Verification items for the finished model (mm, model axes). A direction names the side the tool comes from. Give positions to 0.01 mm unless a question says otherwise; leave off trailing zeros. Write each loop counter-clockwise with the first axis right and the second up, starting at its lowest first coordinate (ties: lowest second). Pieces come first, ordered by that corner, then holes. Notation, with made-up numbers: (35.5, -36) - (43.5, -36) arc R12 ccw to (43.5, -14) - close; hole circle Ø7 at (25.5, 56). An arc over 180 degrees is marked (long way). Answer as a JSON object with one key per item and string values. Group by question number.
Item 1: Sectioned sample at B-B, the plane x = 10. Record the boundary of the cut face in (y, z), and give its area (3 significant figures).
Item 2: Sectioned sample at A-A, the plane y = 14.5. Record the boundary of the cut face in (x, z), and give its area (3 significant figures).
Item 3: Tool access check on faces 1 (the face through (48.26, 23, 3)), 2 (the face through (30, 35, 0)), 3 (the face through (67, 40.894, 18)), 4 (the face through (62, 6.35, 8)). Record the directions out of +Z, -Z, +X, -X, +Y, -Y that give a thin tool (end or side, any length) a straight path to the whole face; none if there is none.
Item 4: Draft check along X on faces 5 (the face through (24, 40.894, 3)), 6 (the face through (2.6, 17.71, 2.58)), 7 (the face through (60.743, 23.645, 8.938)). Enter one of: +X half, -X half, draft (parallel to the pull), parting line (faces both ways), or undercut.
Item 5: Scan lines: line 1 along Y through (x, z) = (68.05, 22.86); line 2 along X through (y, z) = (31, 2); line 3 along X through (y, z) = (6, 5.75). Record each from-to range of solid material in increasing order. Write a range as [from, to].
Item 6: Sectioned sample at D-D, the plane y = 38. Record the boundary of the cut face in (x, z).
Item 7: Sectioned sample at C-C, the plane z = 2.5. Record the boundary of the cut face in (x, y) (3 decimals).
Item 8: Go/stop test with flat-tipped pins: pin 1 (1.5 mm diameter, centred on y = 34.417, z = 22.86, fed in from -X); pin 2 (5 mm diameter, centred on x = 18, z = 6.5, fed in from -Y); pin 3 (4 mm diameter, centred on x = 16.5, z = 5, fed in from +Y). Record where each tip stops, or that it passes through.
```python
from build123d import *

# Parameters (mm, degrees)
SKETCH1_W            = 54.61
SKETCH1_H            = 47.244
SKETCH1_W_2          = 41.91
SKETCH1_H_2          = 21.844
BOSS_EXTRUDE1_DEPTH  = 5.08
SKETCH2_R            = 0.93599
CUT_EXTRUDE1_DEPTH   = 73.388217522
SKETCH10_W           = 14.41958
SKETCH10_H           = 19.49958
SKETCH10_R           = 0.635
BOSS_EXTRUDE4_DEPTH  = 5.08
SKETCH11_R           = 0.635
SKETCH11_W           = 3.302
SKETCH11_H           = 76.2
BOSS_EXTRUDE5_DEPTH  = 5.08
SKETCH12_W           = 60.452
SKETCH12_H           = 6.35
SKETCH12_W_2         = 59.182
CUT_EXTRUDE2_DEPTH   = 95.448366629
SKETCH13_W           = 7.0195552
SKETCH13_H           = 78.993394517
BOSS_EXTRUDE6_DEPTH  = 4.826
FILLET1_R            = 2.54
CUT_EXTRUDE3_DEPTH   = 95.448366629
SKETCH15_W           = 9.078627065
SKETCH15_H           = 34.544
BOSS_EXTRUDE7_DEPTH  = 5.08
SKETCH19_W           = 25.4
SKETCH19_H           = 34.544
BOSS_EXTRUDE9_DEPTH  = 4.7625
SKETCH20_W           = 9.525
SKETCH20_H           = 9.525
BOSS_EXTRUDE10_DEPTH = 9.525
SKETCH21_R           = 0.635
CUT_EXTRUDE4_DEPTH   = 98.23065776
SKETCH22_R           = 0.635
CUT_EXTRUDE5_DEPTH   = 98.23065776
RIB1_REACH           = 80.493
SKETCH24_WALL_W      = 169.76250031
SKETCH24_WALL_H      = 2.54
FILLET2_R            = 1.27


with BuildPart() as part:
    # Sketch1 → Boss-Extrude1 (new body)
    with BuildSketch(Plane.XY):
        with Locations((27.305, 23.622)):
            Rectangle(SKETCH1_W, SKETCH1_H)
        with Locations((27.305, 23.622)):
            Rectangle(SKETCH1_W_2, SKETCH1_H_2, mode=Mode.SUBTRACT)
    extrude(amount=BOSS_EXTRUDE1_DEPTH)

    # Sketch2 → Cut-Extrude1 (cut, through all)
    with BuildSketch(Plane.XY.offset(5.08)):
        with Locations((2.80543, 28.62199)):
            Circle(SKETCH2_R)
        with Locations((2.80543, 18.62201)):
            Circle(SKETCH2_R)
        with Locations((51.80457, 28.62199)):
            Circle(SKETCH2_R)
        with Locations((51.80457, 18.62201)):
            Circle(SKETCH2_R)
    extrude(amount=-CUT_EXTRUDE1_DEPTH, mode=Mode.SUBTRACT)

    # Sketch10 → Boss-Extrude4 (add)
    with BuildSketch(Plane.XY.offset(5.08)):
        with Locations((61.81979, 23.622)):
            Rectangle(SKETCH10_W, SKETCH10_H)
        with Locations((64.35979, 21.49221)):
            Circle(SKETCH10_R, mode=Mode.SUBTRACT)
        with Locations((64.35979, 25.75179)):
            Circle(SKETCH10_R, mode=Mode.SUBTRACT)
    extrude(amount=-BOSS_EXTRUDE4_DEPTH)

    # Sketch11 → Boss-Extrude5 (add)
    with BuildSketch(Plane.XY.offset(5.08)):
        Polygon((0, 47.244), (-5.842, 47.244), (-5.842, 64.262), (-15.748, 64.262), (-15.748, -17.018), (-4.572, -17.018), (-4.572, 0), (0, 0), align=None)
        with Locations(Location((-4.572, 21.49221, 0), (0, 0, 180))):
            Circle(SKETCH11_R, mode=Mode.SUBTRACT)
        with Locations(Location((-4.572, 25.75179, 0), (0, 0, 180))):
            Circle(SKETCH11_R, mode=Mode.SUBTRACT)
        with Locations((-10.795, 23.622)):
            Rectangle(SKETCH11_W, SKETCH11_H, mode=Mode.SUBTRACT)
    extrude(amount=-BOSS_EXTRUDE5_DEPTH)

    # Sketch12 → Cut-Extrude2 (cut, through all)
    with BuildSketch(Plane.XY.offset(5.08)):
        with Locations((24.384, 44.069)):
            Rectangle(SKETCH12_W, SKETCH12_H)
        with Locations((25.019, 3.175)):
            Rectangle(SKETCH12_W_2, SKETCH12_H)
    extrude(amount=-CUT_EXTRUDE2_DEPTH, mode=Mode.SUBTRACT)

    # Sketch13 → Boss-Extrude6 (add)
    with BuildSketch(Plane(origin=(0, 0, 0), x_dir=(-1, 0, 0), z_dir=(0, 0, -1))):
        with Locations((10.665198327, 23.388014827)):
            Rectangle(SKETCH13_W, SKETCH13_H)
    extrude(amount=-BOSS_EXTRUDE6_DEPTH)

    # Fillet1
    fillet1_edges = [part.edges().sort_by_distance(p)[0] for p in [
        (69.02958, 13.87221, 2.54),
        (54.61, 13.87221, 2.54),
        (54.61, 6.35, 2.54),
        (-4.572, 6.35, 2.54),
        (-4.572, -17.018, 2.54),
        (-15.748, -17.018, 2.54),
        (-15.748, 64.262, 2.54),
        (-5.842, 64.262, 2.54),
        (-5.842, 40.894, 2.54),
        (54.61, 40.894, 2.54),
        (54.61, 33.37179, 2.54),
        (69.02958, 33.37179, 2.54),
    ]]
    fillet(fillet1_edges, radius=FILLET1_R)

    # Sketch14 → Cut-Extrude3 (cut, through all)
    with BuildSketch(Plane.XY.offset(5.08)):
        Polygon((2.80543, 40.894), (-0.815942935, 40.894), (-0.815942935, 6.35), (2.80543, 6.35), (2.80543, -19.941776761), (-23.515321153, -19.941776761), (-23.515321153, 65.826532556), (2.80543, 65.826532556), align=None)
        Polygon((51.80457, 40.896870143), (51.80457, 65.826532556), (74.486186006, 65.826532556), (74.486186006, -19.941776761), (51.80457, -19.941776761), (52.07, 6.35), (54.61, 8.89), (54.61, 38.354), align=None)
    extrude(amount=-CUT_EXTRUDE3_DEPTH, mode=Mode.SUBTRACT)

    # Sketch15 → Boss-Extrude7 (add)
    with BuildSketch(Plane.XY.offset(5.08)):
        with Locations((-5.355256468, 23.622)):
            Rectangle(SKETCH15_W, SKETCH15_H)
        Polygon((51.807736495, 40.894), (54.61, 38.354), (54.61, 8.89), (52.07, 6.35), (64.50457, 6.35), (64.50457, 40.894), align=None)
    extrude(amount=-BOSS_EXTRUDE7_DEPTH)

    # Sketch19 → Boss-Extrude9 (add)
    with BuildSketch(Plane(origin=(64.50457, 0, 0), x_dir=(0, 0, -1), z_dir=(1, 0, 0))):
        with Locations((-12.7, 23.622)):
            Rectangle(SKETCH19_W, SKETCH19_H)
    extrude(amount=BOSS_EXTRUDE9_DEPTH)

    # Sketch20 → Boss-Extrude10 (add)
    with BuildSketch(Plane(origin=(69.26707, 0, 0), x_dir=(0, 0, -1), z_dir=(1, 0, 0))):
        with Locations((-4.7625, 45.6565)):
            Rectangle(SKETCH20_W, SKETCH20_H)
        with Locations((-4.7625, 1.5875)):
            Rectangle(SKETCH20_W, SKETCH20_H)
    extrude(amount=-BOSS_EXTRUDE10_DEPTH)

    # Sketch21 → Cut-Extrude4 (cut, through all)
    with BuildSketch(Plane(origin=(69.26707, 0, 0), x_dir=(0, 0, -1), z_dir=(1, 0, 0))):
        with Locations((-4.7625, 45.6565)):
            Circle(SKETCH21_R)
        with Locations((-4.7625, 1.5875)):
            Circle(SKETCH21_R)
    extrude(amount=-CUT_EXTRUDE4_DEPTH, mode=Mode.SUBTRACT)

    # Sketch22 → Cut-Extrude5 (cut, through all)
    with BuildSketch(Plane(origin=(69.26707, 0, 0), x_dir=(0, 0, -1), z_dir=(1, 0, 0))):
        with Locations((-22.86, 34.417)):
            Circle(SKETCH22_R)
        with Locations((-22.86, 12.827)):
            Circle(SKETCH22_R)
        with Locations((-16.51, 34.417)):
            Circle(SKETCH22_R)
        with Locations((-10.16, 34.417)):
            Circle(SKETCH22_R)
        with Locations((-10.16, 12.827)):
            Circle(SKETCH22_R)
        with Locations((-16.51, 12.827)):
            Circle(SKETCH22_R)
    extrude(amount=-CUT_EXTRUDE5_DEPTH, mode=Mode.SUBTRACT)

    # Sketch24 wall → Rib1 (add, up to next)
    with BuildSketch(Plane(origin=(60.69457, 23.622, 8.89), x_dir=(-0.707106781187, 0, -0.707106781187), z_dir=(0.707106781187, 0, -0.707106781187)), mode=Mode.PRIVATE) as rib1_sk1:
        Rectangle(SKETCH24_WALL_W, SKETCH24_WALL_H)
    rib1_tool1 = extrude(rib1_sk1.sketch, amount=RIB1_REACH, mode=Mode.PRIVATE) - part.part
    add(rib1_tool1.solids().sort_by_distance((60.69457, 23.622, 8.89))[0])

    # Fillet2
    fillet2_edges = [part.edges().sort_by_distance(p)[0] for p in [
        (62.12332, 6.35, 5.08),
        (64.50457, 14.351, 5.08),
        (66.88582, 40.894, 25.4),
        (66.88582, 6.35, 25.4),
        (62.12332, 40.894, 5.08),
        (66.88582, 40.894, 9.525),
        (66.88582, 6.35, 9.525),
        (64.50457, 32.893, 5.08),
        (64.50457, 23.622, 12.7),
        (56.88457, 23.622, 5.08),
        (60.69457, 22.352, 5.08),
        (60.69457, 24.892, 5.08),
    ]]
    fillet(fillet2_edges, radius=FILLET2_R)


solid = part.part
```
Geometry check:
{
 "1": {"outline": "(6.35, 0) - (12.7, 0) - (12.7, 5.08) - (6.35, 5.08) - close; (34.54, 0) - (40.89, 0) - (40.89, 5.08) - (34.54, 5.08) - close", "area": "64.5 mm^2"},
 "2": {"outline": "(-9.89, 0) - (6.35, 0) - (6.35, 5.08) - (-9.89, 5.08) - close; (48.26, 0) - (69.27, 0) - (69.27, 25.4) - (64.5, 25.4) - (64.5, 6.35) arc R1.27 cw to (63.23, 5.08) - (48.26, 5.08) - close", "area": "286 mm^2"},
 "3": {"face 1": "+Z, -Z", "face 2": "-Z, +X, -X, +Y, -Y", "face 3": "+Z, +X, -X, +Y", "face 4": "+Z, -X"},
 "4": {"face 5": "draft", "face 6": "undercut", "face 7": "-X half"},
 "5": {"line 1": "[6.35, 12.19], [13.46, 33.78], [35.05, 40.89]", "line 2": "[-9.89, 6.35], [48.26, 69.27]", "line 3": "[59.74, 69.27]"},
 "6": {"outline": "(-9.89, 0) - (69.27, 0) - (69.27, 25.4) - (64.5, 25.4) - (64.5, 6.35) arc R1.27 cw to (63.23, 5.08) - (-9.89, 5.08) - close"},
 "7": {"outline": "(-9.895, 6.35) - (59.742, 6.35) - (59.742, -3.175) - (69.267, -3.175) - (69.267, 50.419) - (59.742, 50.419) - (59.742, 40.894) - (-9.895, 40.894) - close; hole circle Ø1.872 at (2.805, 18.622); hole circle Ø1.872 at (2.805, 28.622); hole (6.35, 12.7) - (48.26, 12.7) - (48.26, 34.544) - (6.35, 34.544) - close; hole circle Ø1.872 at (51.805, 18.622); hole circle Ø1.872 at (51.805, 28.622)"},
 "8": {"pin 1": "x = 64.5", "pin 2": "y = 6.35", "pin 3": "y = 40.89"}
}
